Verification items for the finished model (mm, model axes). A direction names the side the tool comes from. Round coordinates to 2 decimals unless told otherwise and drop trailing zeros. Write each loop counter-clockwise with the first axis right and the second up, starting at its lowest first coordinate (ties: lowest second). Pieces come first, ordered by that corner, then holes. Notation, with made-up numbers: M -23,63 L 30,63 A24 ccw 30,98 Z; hole C 45,36 d5. An arc over 180 degrees is marked long. One line per question, with ' | ' between items. Start each with the question number.
Q1. Cross-section at B-B (x = 63.5). Record the boundary of the cut face in (y, z) (3 decimals).
Q2. Cross-section at C-C (y = -106). Record the boundary of the cut face in (x, z) (3 decimals), then the cut area to 3 significant figures.
Q3. Tool access check on faces 4 (the face through (63.291, -64.389, 3.177)), 5 (the face through (0, -63, 63)). Record the directions out of +Z, -Z, +X, -X, +Y, -Y that give a thin tool (end or side, any length) a straight path to the whole face; none if there is none.
Q4. Cross-section at D-D (x = 118). Record the boundary of the cut face in (y, z).
Q5. Cross-section at A-A (z = 16.5). Record the boundary of the cut face in (x, y) (3 decimals), then the cut area to 3 significant figures.
Q6. Gauge pin test, flat ends, axial feed: pin 1 (8 mm diameter, centred on y = -38, z = 56, fed in from +X); pin 2 (2 mm diameter, centred on x = 93.5, y = -92.5, fed in from +Z). Record the tip position at first contact, or that the pin passes through.
Q7. Release check for a two-part mould opening along X. For faces 1 (the face through (108.2, -62.6, 88.4)), 2 (the face through (73.025, -64, 63)), 3 (the face through (44, -63, 127)) record: released by +X, released by -X, zero draft, split by the parting line, or undercut.
Q8. Thickness scan on line 1 along X through (y, z) = (-91, 27) (3 decimals); line 2 along X through (y, z) = (-59.5, 75) (3 decimals); line 3 along Z through (x, y) = (58.5, -109.5). Record the ranges inside material, lowest first. Write a range as from..to.
from build123d import *

# Parameters (mm, degrees)
F0_W     = 127
F0_H     = 127
F1_DEPTH = 127
F3_DEPTH = 127
F4_SIZE2 = 76.2
F4_SIZE  = 38.1


with BuildPart() as f1:
    # F0 (on Front) → F1 (new body)
    with BuildSketch(Plane.XZ):
        with Locations((63.5, 63.5)):
            Rectangle(F0_W, F0_H)
    extrude(amount=F1_DEPTH)

    # F2 (on face) → F3 (cut, through all)
    with BuildSketch(Plane.XZ.offset(127)):
        with BuildLine():
            Line((73.025, 12.7), (73.025, 114.3))
            ThreePointArc((73.025, 114.3), (63.5, 123.825), (53.975, 114.3))
            Line((53.975, 114.3), (53.975, 12.7))
            ThreePointArc((53.975, 12.7), (63.5, 3.175), (73.025, 12.7))
        make_face()
    extrude(amount=-F3_DEPTH, mode=Mode.SUBTRACT)

    # F4
    f4_edges = [f1.edges().sort_by_distance(p)[0] for p in [
        (127, -63.5, 127),
    ]]
    chamfer(f4_edges, length=F4_SIZE, length2=F4_SIZE2)


solid = f1.part
Determined:
1) outline: M -127,0 L 0,0 L 0,3.175 L -127,3.175 Z; M -127,123.825 L 0,123.825 L 0,127 L -127,127 Z
2) outline: M 0,0 L 127,0 L 127,50.8 L 88.9,127 L 0,127 Z; hole M 53.975,12.7 A9.525 ccw 73.025,12.7 L 73.025,114.3 A9.525 ccw 53.975,114.3 Z | area: 12,500 mm²
3) face 4: +Y, -Y | face 5: +Z, -Z, -X, +Y, -Y
4) outline: M -127,0 L 0,0 L 0,68.8 L -127,68.8 Z
5) outline: M 0,-127 L 53.975,-127 L 53.975,0 L 0,0 Z; M 73.025,-127 L 127,-127 L 127,0 L 73.025,0 Z | area: 13,700 mm²
6) pin 1: stops at x = 126.4 | pin 2: stops at z = 119.8
7) face 1: released by +X | face 2: undercut | face 3: zero draft
8) line 1: x = 0..53.975, 73.025..127 | line 2: x = 0..53.975, 73.025..114.9 | line 3: z = 0..4.59, 122.41..127
